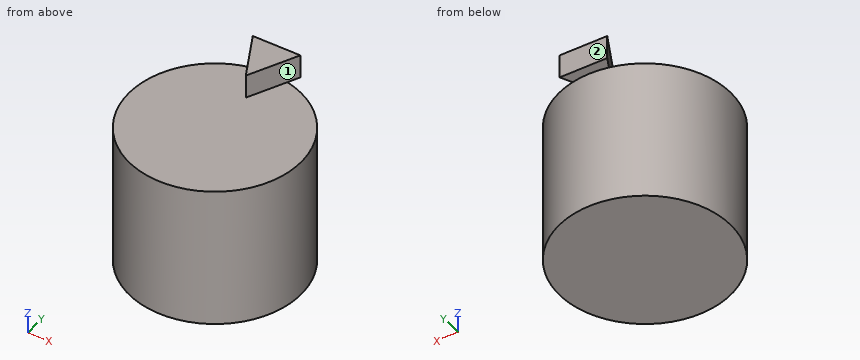
from build123d import *

# Parameters (mm, degrees)
SKETCH1_R           = 36.055512755
BOSS_EXTRUDE1_DEPTH = 60
BOSS_EXTRUDE2_DEPTH = 10


with BuildPart() as part:
    # Sketch1 → Boss-Extrude1 (new body)
    with BuildSketch(Plane.XY):
        with Locations(Location((0, 0, 0), (0, 0, 180))):
            Circle(SKETCH1_R)
    extrude(amount=BOSS_EXTRUDE1_DEPTH)

    # Sketch3 → Boss-Extrude2 (add)
    with BuildSketch(Plane.XY.offset(60)):
        Polygon((-10, 40), (0, 20), (10, 40), align=None)
    extrude(amount=BOSS_EXTRUDE2_DEPTH)


solid = part.part
Work out the finished part from the listing and answer in its coordinate system (mm). Face numbers are marked on the shaded views. A direction names the side the tool comes from. Give positions to 0.01 mm unless a question says otherwise; leave off trailing zeros. Order: outer loops, then holes, each group sorted by start corner. A loop starts at its lowest first (then second) coordinate and runs counter-clockwise, first axis right, second up. Notation, with made-up numbers: M 84.5,-26.75 L 108.5,-26.75 A32 cw 108.5,10.25 Z; hole C 40.25,68.5 d6. An arc over 180 degrees is marked long. Return JSON: item names as keys, results as strings.
Q1. Each of these flat-tipped pins is pushed along its axis until it touches: pin 1 (12 mm diameter, centred on y = 13, z = 35.5, fed in from -X); pin 2 (2 mm diameter, centred on y = 5.5, z = 37, fed in from -X); pin 3 (8 mm diameter, centred on y = -7.5, z = 18.5, fed in from -X). Where does it stop, or does it pass through?
Answer below:
{"pin 1": "stops at x = -35.37", "pin 2": "stops at x = -35.77", "pin 3": "stops at x = -35.89"}
Q2. Find section C-C, the plane x = -31. Write down the section's boundary in (y, z), and give its area (3 significant figures).
Answer below:
{"outline": "M -18.41,0 L 18.41,0 L 18.41,60 L -18.41,60 Z", "area": "2,210 mm^2"}
Q3. Find the intervals of material crossed by line 1 along Z through (x, y) = (8, 13); line 2 along Y through (x, z) = (-28.5, 10.5); line 3 along X through (y, z) = (18, 51), in increasing order. Write a range as [from, to].
Answer below:
{"line 1": "z = [0, 60]", "line 2": "y = [-22.09, 22.09]", "line 3": "x = [-31.24, 31.24]"}
Q4. Find section D-D, the plane y = 0. Write down the section's boundary in (x, z), and give its area (3 significant figures).
Answer below:
{"outline": "M -36.06,0 L 36.06,0 L 36.06,60 L -36.06,60 Z", "area": "4,330 mm^2"}
Q5. Which of the six approach directions +Z, -Z, +X, -X, +Y, -Y give full straight-line access (tool end or side, diameter ignored) to the marked faces 1 and 2?
Answer below:
{"face 1": "+Z, +X, -Y", "face 2": "+Z, -Z, +X, -X, +Y"}
Q6. Find section A-A, the plane y = 30. Write down the section's boundary in (x, z).
Answer below:
{"outline": "M -20,0 L 20,0 L 20,60 L 5,60 L 5,70 L -5,70 L -5,60 L -20,60 Z"}
Q7. Find section B-B, the plane z = 47. Write down the section's boundary in (x, y).
Answer below:
{"outline": "C 0,0 d72.11"}
